```python
from build123d import *

# Parameters (mm, degrees)
SKETCH1_W         = 210
SKETCH1_H         = 210
MAINEXTRUDE_DEPTH = 1
SKETCH1_6_R       = 1.5
SCREWHOLES_DEPTH  = 1
ROUNDEDCORNERS_R  = 10
TRENCH_DEPTH      = 12


with BuildPart() as part:
    # Sketch1 → MainExtrude (new body)
    with BuildSketch(Plane(origin=(0, 0, 0), x_dir=(1, 0, 0), z_dir=(0, 1, 0))):
        Rectangle(SKETCH1_W, SKETCH1_H)
    extrude(amount=MAINEXTRUDE_DEPTH)

    # Sketch1<6> → ScrewHoles (cut)
    with BuildSketch(Plane(origin=(0, 0, 0), x_dir=(1, 0, 0), z_dir=(0, 1, 0))):
        with Locations(Location((-99.833273811, 99.833273811, 0), (0, 0, 270))):
            Circle(SKETCH1_6_R)
        with Locations(Location((-99.833273811, -99.833273811, 0), (0, 0, 90))):
            Circle(SKETCH1_6_R)
        with Locations(Location((99.833273811, -99.833273811, 0), (0, 0, 270))):
            Circle(SKETCH1_6_R)
        with Locations(Location((99.833273811, 99.833273811, 0), (0, 0, 90))):
            Circle(SKETCH1_6_R)
    extrude(amount=SCREWHOLES_DEPTH, mode=Mode.SUBTRACT)

    # RoundedCorners
    roundedcorners_edges = [part.edges().sort_by_distance(p)[0] for p in [
        (-105, 0.5, -105),
        (-105, 0.5, 105),
        (105, 0.5, 105),
        (105, 0.5, -105),
    ]]
    fillet(roundedcorners_edges, radius=ROUNDEDCORNERS_R)

    # Sketch3 → Trench (cut)
    with BuildSketch(Plane(origin=(0, 0, 0), x_dir=(1, 0, 0), z_dir=(0, 1, 0))):
        Polygon((-57, 93), (-57, 33), (-93, 33), (-93, 23), (57, 23), (57, -43), (-83, -43), (-83, -13), (37, -13), (37, -3), (-93, -3), (-93, -53), (-27, -53), (-27, -93), (93, -93), (93, 87), (-27, 87), (-27, 77), (83, 77), (83, -83), (-17, -83), (-17, -53), (67, -53), (67, 33), (-47, 33), (-47, 93), align=None)
    extrude(amount=TRENCH_DEPTH, mode=Mode.SUBTRACT)


solid = part.part
```
Build history of the part. All positions in model axes, mm. Coordinates: 2 decimals unless noted, no trailing zeros. Order: outer loops, then holes, each group sorted by start corner. A loop starts at its lowest first (then second) coordinate and runs counter-clockwise, first axis right, second up.
Item 1: Saw through at D-D on z = 34. List the corners of the cut face in (x, y).
Filled in:
outline: (-105, 0) - (-93, 0) - (-93, 1) - (-105, 1) - close; (-83, 0) - (57, 0) - (57, 1) - (-83, 1) - close; (67, 0) - (83, 0) - (83, 1) - (67, 1) - close; (93, 0) - (105, 0) - (105, 1) - (93, 1) - close
Item 2: Drill centre lines: L1, parallel to X at y = 0.25, z = -64.5; L2, parallel to X at y = 0.3, z = 70; L3, parallel to Z at x = 35, y = 0.95. Where is each one in solid material? Low to high.
Filled in:
L1: x = -105 to -57, -47 to 83, 93 to 105
L2: x = -105 to -27, -17 to 83, 93 to 105
L3: z = -105 to -87, -77 to -33, -23 to 3, 13 to 43, 53 to 83, 93 to 105
Item 3: Saw through at B-B on z = -28. List the corners of the cut face in (x, y).
Filled in:
outline: (-105, 0) - (-93, 0) - (-93, 1) - (-105, 1) - close; (67, 0) - (83, 0) - (83, 1) - (67, 1) - close; (93, 0) - (105, 0) - (105, 1) - (93, 1) - close
Item 4: Saw through at C-C on x = 63. List the corners of the cut face in (y, z), then the cut area to 3 significant figures.
Filled in:
outline: (0, -105) - (1, -105) - (1, -87) - (0, -87) - close; (0, -77) - (1, -77) - (1, -33) - (0, -33) - close; (0, 53) - (1, 53) - (1, 83) - (0, 83) - close; (0, 93) - (1, 93) - (1, 105) - (0, 105) - close
area: 104 mm2
Item 5: Saw through at A-A on x = -87.5. List the corners of the cut face in (y, z).
Filled in:
outline: (0, -105) - (1, -105) - (1, -33) - (0, -33) - close; (0, -23) - (1, -23) - (1, 3) - (0, 3) - close; (0, 53) - (1, 53) - (1, 105) - (0, 105) - close
